Input: part model. Units: mm. Frame: model coordinates. A direction names the side the tool comes from. Round coordinates to 2 decimals unless told otherwise and drop trailing zeros. Loops run counter-clockwise (first coordinate to the right, second up) from the corner with the lowest first, then second, coordinate; pieces in that order, holes last.
(1) First-contact query: pin 1 Ø2 at (x, y) = (31, 1) entering from +Z. Flat tip, straight axial feed; report the tip coordinate or a pass-through.
(2) Draft query along Y for faces 3 (the face through (81, 3, 12)), 4 (the face through (4.133, 1.095, 10.986)), 5 (the face through (6.386, 4.425, 5.916)). Return one class per face: released by +Y, released by -Y, zero draft, split by the parting line, or undercut.
(3) Access query for faces 1 (the face through (77, 5, 11)), 2 (the face through (47, 0, 5)). Directions: +Z, -Z, +X, -X, +Y, -Y. A direction counts if a zero-diameter tool reaches every point of the face in a straight line with its end or side. Return the directions, or none.
(4) Cut plane A-A, the plane x = 5. Output: boundary loops of the cut face in (y, z).
(5) Line query: line 1 (Y direction, x = 91, z = 7); line 2 (Z direction, x = 61, y = 5); line 3 (Y direction, x = 14, z = 4.75). Output: solid intervals per line, ascending.
(6) Cut plane D-D, the plane x = 15. Output: boundary loops of the cut face in (y, z), and give its area (3 significant figures).
(7) Cut plane B-B, the plane y = 5. Output: boundary loops of the cut face in (x, z), and give its area (3 significant figures).
(8) Cut plane C-C, the plane z = 3. Output: boundary loops of the cut face in (x, y), and give its area (3 significant figures).
from build123d import *

# Parameters (mm, degrees)
SKETCH_W      = 95
SKETCH_H      = 10
SKETCH_R      = 1.5
PAD_DEPTH     = 10
SKETCH001_R   = 4
SKETCH001_R_2 = 1.5
PAD001_DEPTH  = 2


with BuildPart() as part:
    # Sketch → Pad (new body)
    with BuildSketch(Plane.XY):
        with Locations((47.5, 5)):
            Rectangle(SKETCH_W, SKETCH_H)
        with Locations((5, 5)):
            Circle(SKETCH_R, mode=Mode.SUBTRACT)
        with Locations((81, 5)):
            Circle(SKETCH_R, mode=Mode.SUBTRACT)
        with Locations((91, 5)):
            Circle(SKETCH_R, mode=Mode.SUBTRACT)
        with Locations((15, 5)):
            Circle(SKETCH_R, mode=Mode.SUBTRACT)
    extrude(amount=PAD_DEPTH)

    # Sketch001 (on Face10 of Pad) → Pad001 (join)
    with BuildSketch(Plane.XY.offset(10)):
        with Locations((5, 5)):
            Circle(SKETCH001_R)
        with Locations((5, 5)):
            Circle(SKETCH001_R_2, mode=Mode.SUBTRACT)
        with Locations((81, 5)):
            Circle(SKETCH001_R)
        with Locations((81, 5)):
            Circle(SKETCH001_R_2, mode=Mode.SUBTRACT)
    extrude(amount=PAD001_DEPTH)


solid = part.part
Reported:
1. pin 1: stops at z = 10
2. face 3: zero draft
2. face 4: split by the parting line
2. face 5: undercut
3. face 1: +Z
3. face 2: +Z, -Z, +X, -X, -Y
4. outline: (0, 0) - (3.5, 0) - (3.5, 12) - (1, 12) - (1, 10) - (0, 10) - close; (6.5, 0) - (10, 0) - (10, 10) - (9, 10) - (9, 12) - (6.5, 12) - close
5. line 1: y = 0 to 3.5, 6.5 to 10
5. line 2: z = 0 to 10
5. line 3: y = 0 to 3.88, 6.12 to 10
6. outline: (0, 0) - (3.5, 0) - (3.5, 10) - (0, 10) - close; (6.5, 0) - (10, 0) - (10, 10) - (6.5, 10) - close
6. area: 70.0 mm2
7. outline: (0, 0) - (3.5, 0) - (3.5, 12) - (1, 12) - (1, 10) - (0, 10) - close; (6.5, 0) - (13.5, 0) - (13.5, 10) - (9, 10) - (9, 12) - (6.5, 12) - close; (16.5, 0) - (79.5, 0) - (79.5, 12) - (77, 12) - (77, 10) - (16.5, 10) - close; (82.5, 0) - (89.5, 0) - (89.5, 10) - (85, 10) - (85, 12) - (82.5, 12) - close; (92.5, 0) - (95, 0) - (95, 10) - (92.5, 10) - close
7. area: 850 mm2
8. outline: (0, 0) - (95, 0) - (95, 10) - (0, 10) - close; hole circle Ø3 at (5, 5); hole circle Ø3 at (15, 5); hole circle Ø3 at (81, 5); hole circle Ø3 at (91, 5)
8. area: 922 mm2
